The figure shows three views and two pictorial views of one solid part (mm, origin at its lowest corner). Answer the questions. A direction names the side the tool comes from. Round coordinates to 2 decimals unless told otherwise and drop trailing zeros. Order: outer loops, then holes, each group sorted by start corner. A loop starts at its lowest first (then second) coordinate and runs counter-clockwise, first axis right, second up. Notation, with made-up numbers: (81.5, 85.25) - (102.5, 85.25) arc R16 cw to (102.5, 102.25) - close; hole circle Ø10 at (-36, 73). An arc over 180 degrees is marked (long way). Write item = value, one per line.
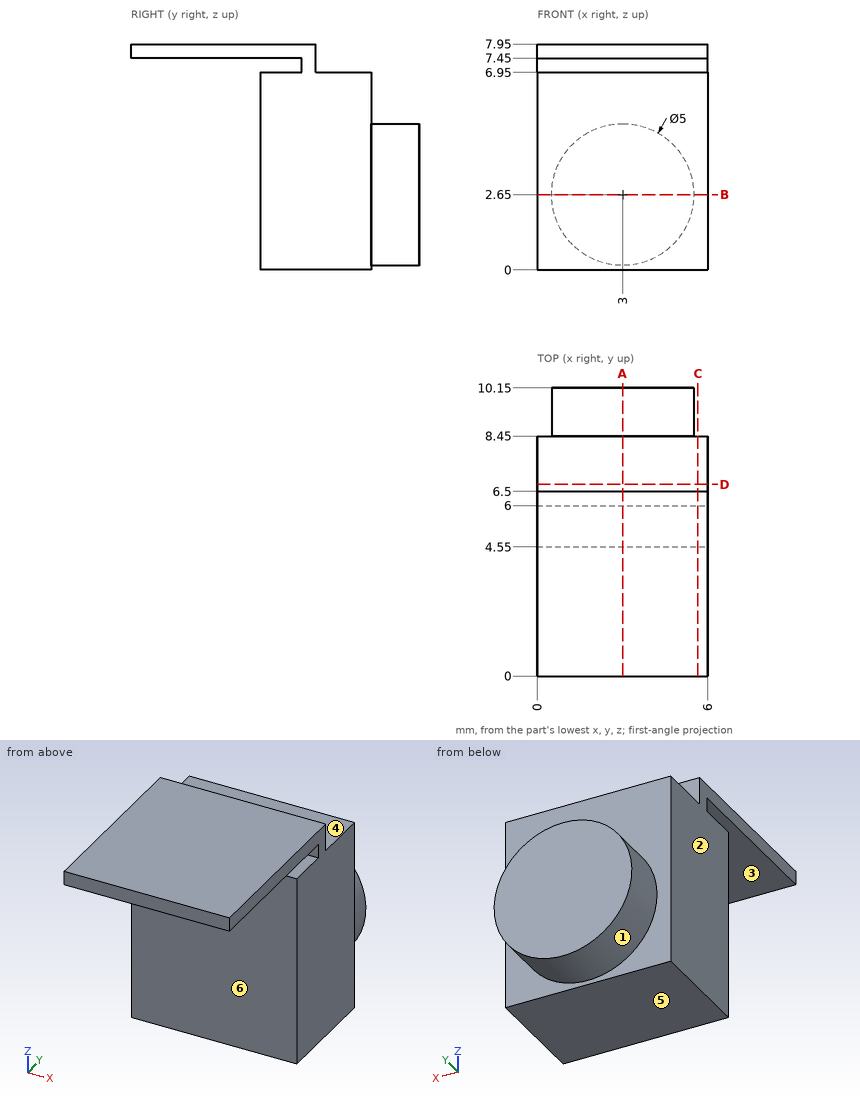
Q1. Section D-D on y = 6.75 is taken. Determine the outline of the cut face in (x, z), then the cut area to 3 significant figures.
Model answer:
outline = (0, 0) - (6, 0) - (6, 6.95) - (0, 6.95) - close
area = 41.7 mm^2
Q2. Flat-ended cylindrical pins translate along their axes: P1, Ø0.5, axis at x = 4, z = 7.5, coming from the +Y side; P2, Ø3, axis at x = 1, z = 2.5, coming from the -Y side; P3, Ø1, axis at x = 4, y = 7.5, coming from the +Z side. Find the tip coordinate at first contact, or state that the pin passes through.
Model answer:
P1 = 6.5
P2 = 4.55
P3 = 6.95
Q3. Section A-A on x = 3 is taken. Determine the outline of the cut face in (y, z), then the cut area to 3 significant figures.
Model answer:
outline = (0, 7.45) - (6, 7.45) - (6, 6.95) - (4.55, 6.95) - (4.55, 0) - (8.45, 0) - (8.45, 0.15) - (10.15, 0.15) - (10.15, 5.15) - (8.45, 5.15) - (8.45, 6.95) - (6.5, 6.95) - (6.5, 7.95) - (0, 7.95) - close
area = 39.1 mm^2
Q4. Determine the mould class of the marked faces 1, 2 and 3 for opening direction Z: released by +Z, released by -Z, zero draft, split by the parting line, or undercut.
Model answer:
face_1 = split by the parting line
face_2 = zero draft
face_3 = undercut
Q5. For the marked faces 4, 5 and 6, determine the directions among +Z, -Z, +X, -X, +Y, -Y from which every point of the face is accessible in a straight line to the end or side of a thin tool.
Model answer:
face_4 = +Z, +X, -X, +Y
face_5 = -Z, +X, -X, +Y, -Y
face_6 = -Z, +X, -X, -Y
Q6. Find the intervals of material crossed by line 1 (Z direction, x = 1.5, y = 4.75); line 2 (Y direction, x = 4.5, z = 2.25); line 3 (Z direction, x = 0.45, y = 3), in increasing order. Write a range as from..to.
Model answer:
line_1 = 0..6.95, 7.45..7.95
line_2 = 4.55..10.15
line_3 = 7.45..7.95
Q7. Section C-C on x = 5.65 is taken. Determine the outline of the cut face in (y, z), then the cut area to 3 significant figures.
Model answer:
outline = (0, 7.45) - (6, 7.45) - (6, 6.95) - (4.55, 6.95) - (4.55, 0) - (8.45, 0) - (8.45, 6.95) - (6.5, 6.95) - (6.5, 7.95) - (0, 7.95) - close
area = 30.6 mm^2
Q8. Section B-B on z = 2.65 is taken. Determine the outline of the cut face in (x, y), then the cut area to 3 significant figures.
Model answer:
outline = (0, 4.55) - (6, 4.55) - (6, 8.45) - (5.5, 8.45) - (5.5, 10.15) - (0.5, 10.15) - (0.5, 8.45) - (0, 8.45) - close
area = 31.9 mm^2
